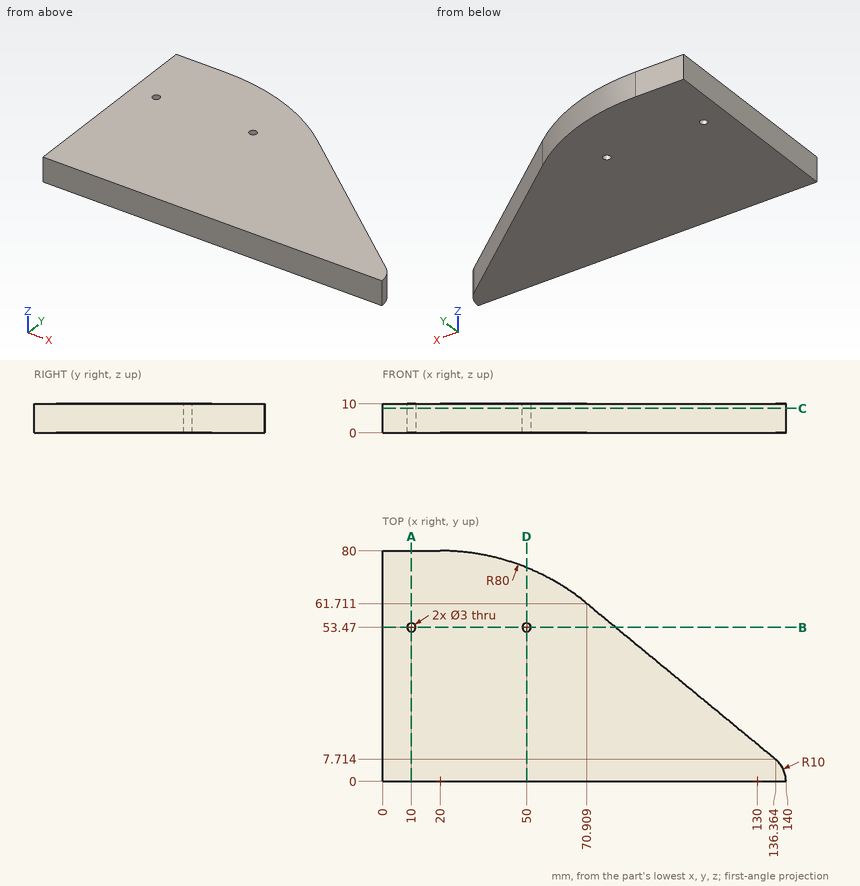
Here's the drawing with two shaded views (mm, measured from the low corner). I have some questions. Coordinates: 2 decimals unless noted, no trailing zeros. Write each loop counter-clockwise with the first axis right and the second up, starting at its lowest first coordinate (ties: lowest second). Pieces come first, ordered by that corner, then holes.
Item 1: If I drill on line 1 (Y direction, x = 50, z = 3); line 2 (Y direction, x = 110, z = 4); line 3 (X direction, y = 22.5, z = 7), over which ranges is the centre line in solid material (lowest first)?
Item 2: I want a section at C-C on z = 8.5. Write out the boundary of the cut face in (x, y), and give its area (3 significant figures).
Item 3: I want a section at D-D on x = 50. Write out the boundary of the cut face in (y, z).
Item 4: I want a section at A-A on x = 10. Write out the boundary of the cut face in (y, z), and give its area (3 significant figures).
Item 5: I want a section at B-B on y = 53.47. Write out the boundary of the cut face in (x, z).
Item 6: Will these pins go through, and if not, where does the flat tip stop? pin 1 (1.5 mm diameter, centred on y = 24, z = 4, fed in from +X); pin 2 (1 mm diameter, centred on y = 18.5, z = 1.5, fed in from +X) (1 decimal); pin 3 (2.5 mm diameter, centred on x = 50, y = 53.47, fed in from +Z); pin 4 (4 mm diameter, centred on y = 16, z = 2.5, fed in from +X) (1 decimal).
Findings below:
1. line 1: y = 0 to 51.97, 54.97 to 74.16
1. line 2: y = 0 to 29.46
1. line 3: x = 0 to 118.44
2. outline: (0, 0) - (140, 0) arc R10 ccw to (136.36, 7.71) - (70.91, 61.71) arc R80 ccw to (20, 80) - (0, 80) - close; hole circle Ø3 at (10, 53.47); hole circle Ø3 at (50, 53.47)
2. area: 7,660 mm2
3. outline: (0, 0) - (51.97, 0) - (51.97, 10) - (0, 10) - close; (54.97, 0) - (74.16, 0) - (74.16, 10) - (54.97, 10) - close
4. outline: (0, 0) - (51.97, 0) - (51.97, 10) - (0, 10) - close; (54.97, 0) - (80, 0) - (80, 10) - (54.97, 10) - close
4. area: 770 mm2
5. outline: (0, 0) - (8.5, 0) - (8.5, 10) - (0, 10) - close; (11.5, 0) - (48.5, 0) - (48.5, 10) - (11.5, 10) - close; (51.5, 0) - (80.9, 0) - (80.9, 10) - (51.5, 10) - close
6. pin 1: stops at x = 117.53
6. pin 2: stops at x = 123.9
6. pin 3: passes through
6. pin 4: stops at x = 128.7
